```python
from build123d import *

# Parameters (mm, degrees)
LID_BLANK_DEPTH                 = 56
OUTER_PANEL_20DEG_DEPTH         = 143.098557347
OUTER_PANEL_20DEG_DEPTH_BACK    = 143.098557347
PANEL_3MM_DEPTH                 = 141.483885809
PANEL_3MM_DEPTH_BACK            = 141.483885809
HIDDEN_CASE_POST_0_START        = 3
SKETCH_4_R                      = 5
HIDDEN_CASE_POST_0_DEPTH        = 22.878191011
HIDDEN_CASE_POST_1_START        = 3
SKETCH_5_R                      = 5
HIDDEN_CASE_POST_1_DEPTH        = 22.878191011
HIDDEN_CASE_POST_2_START        = 3
SKETCH_6_R                      = 5
HIDDEN_CASE_POST_2_DEPTH        = 48.720077644
HIDDEN_CASE_POST_3_START        = 3
SKETCH_7_R                      = 5
HIDDEN_CASE_POST_3_DEPTH        = 48.720077644
FLUSH_OUTER_SURFACE_DEPTH       = 141.483885809
FLUSH_OUTER_SURFACE_DEPTH_BACK  = 141.483885809
BLIND_M3_0_START                = 3
SKETCH_9_R                      = 1.7
BLIND_M3_0_DEPTH                = 9.5
M3_SIDE_LOAD_NUT_0_START        = 3.1
SKETCH_10_W                     = 2.8
SKETCH_10_H                     = 5.8
M3_SIDE_LOAD_NUT_0_DEPTH        = 9.4
BLIND_M3_1_START                = 3
SKETCH_11_R                     = 1.7
BLIND_M3_1_DEPTH                = 9.5
M3_SIDE_LOAD_NUT_1_START        = 87.5
SKETCH_12_W                     = 2.8
SKETCH_12_H                     = 5.8
M3_SIDE_LOAD_NUT_1_DEPTH        = 9.4
BLIND_M3_2_START                = 3
SKETCH_13_R                     = 1.7
BLIND_M3_2_DEPTH                = 9.5
M3_SIDE_LOAD_NUT_2_START        = 3.1
SKETCH_14_W                     = 2.8
SKETCH_14_H                     = 5.8
M3_SIDE_LOAD_NUT_2_DEPTH        = 9.4
BLIND_M3_3_START                = 3
SKETCH_15_R                     = 1.7
BLIND_M3_3_DEPTH                = 9.5
M3_SIDE_LOAD_NUT_3_START        = 87.5
SKETCH_16_W                     = 2.8
SKETCH_16_H                     = 5.8
M3_SIDE_LOAD_NUT_3_DEPTH        = 9.4
SKETCH_17_R                     = 4.1
SHAFT_D8P2_DEPTH                = 5
SKETCH_18_W                     = 13.3
SKETCH_18_H                     = 13.3
BUTTON_13P3_CLEARANCE_DEPTH     = 5
SKETCH_19_R                     = 4
ENCODER_FRONT_BLIND_POST_DEPTH  = 11.07
ENCODER_FRONT_BLIND_SCREW_START = -14.07
SKETCH_20_R                     = 1.15
ENCODER_FRONT_BLIND_SCREW_DEPTH = 5
ENCODER_FRONT_M2_SIDE_NUT_START = 20.5
ENCODER_FRONT_M2_SIDE_NUT_DEPTH = 7.5
SKETCH_22_R                     = 4
ENCODER_REAR_BLIND_POST_DEPTH   = 11.07
ENCODER_REAR_BLIND_SCREW_START  = -14.07
SKETCH_23_R                     = 1.15
ENCODER_REAR_BLIND_SCREW_DEPTH  = 5
ENCODER_REAR_M2_SIDE_NUT_START  = 44.5
ENCODER_REAR_M2_SIDE_NUT_DEPTH  = 7.5
SKETCH_25_R                     = 4
BUTTON_LEFT_BLIND_POST_DEPTH    = 6.7
BUTTON_LEFT_BLIND_SCREW_START   = -9.7
SKETCH_26_R                     = 1.15
BUTTON_LEFT_BLIND_SCREW_DEPTH   = 5
BUTTON_LEFT_M2_SIDE_NUT_START   = 57.5
BUTTON_LEFT_M2_SIDE_NUT_DEPTH   = 7.5
SKETCH_28_R                     = 3.4
BUTTON_RIGHT_BLIND_POST_DEPTH   = 6.7
BUTTON_RIGHT_BLIND_SCREW_START  = -9.7
SKETCH_29_R                     = 1.15
BUTTON_RIGHT_BLIND_SCREW_DEPTH  = 5
BUTTON_RIGHT_M2_SIDE_NUT_START  = 90.8
BUTTON_RIGHT_M2_SIDE_NUT_DEPTH  = 7.5


with BuildPart() as part:
    # 草图1 → Lid_blank (new body)
    with BuildSketch(Plane.XY):
        with BuildLine():
            Line((6, 0), (94, 0))
            ThreePointArc((94, 0), (98.242640687, 1.757359313), (100, 6))
            Line((100, 6), (100, 78))
            ThreePointArc((100, 78), (98.242640687, 82.242640687), (94, 84))
            Line((94, 84), (6, 84))
            ThreePointArc((6, 84), (1.757359313, 82.242640687), (0, 78))
            Line((0, 78), (0, 6))
            ThreePointArc((0, 6), (1.757359313, 1.757359313), (6, 0))
        make_face()
    extrude(amount=LID_BLANK_DEPTH)

    # 草图2 → Outer_panel_20deg (cut, two sides: drawn at the far end of the back side and taken through both)
    with BuildSketch(Plane(origin=(0, 0, 0), x_dir=(0, 0, -1), z_dir=(1, 0, 0)).offset(-OUTER_PANEL_20DEG_DEPTH_BACK)):
        Polygon((-13.913128632, -20), (-61.229259087, 110), (-120, 110), (-120, -20), align=None)
    extrude(amount=OUTER_PANEL_20DEG_DEPTH + OUTER_PANEL_20DEG_DEPTH_BACK, mode=Mode.SUBTRACT)

    # 草图3 → Panel_3mm (cut, two sides: drawn at the far end of the back side and taken through both)
    with BuildSketch(Plane(origin=(0, 0, 0), x_dir=(0, 0, -1), z_dir=(1, 0, 0)).offset(-PANEL_3MM_DEPTH_BACK)):
        Polygon((-10.720595315, -20), (-58.036725769, 110), (30, 110), (30, -20), align=None)
    extrude(amount=PANEL_3MM_DEPTH + PANEL_3MM_DEPTH_BACK, mode=Mode.SUBTRACT)

    # 草图4 → Hidden_case_post_0 (add)
    with BuildSketch(Plane.XY.offset(HIDDEN_CASE_POST_0_START)):
        with Locations(Location((6.5, 6.5, 0), (0, 0, 270))):
            Circle(SKETCH_4_R)
    extrude(amount=HIDDEN_CASE_POST_0_DEPTH)

    # 草图5 → Hidden_case_post_1 (add)
    with BuildSketch(Plane.XY.offset(HIDDEN_CASE_POST_1_START)):
        with Locations(Location((93.5, 6.5, 0), (0, 0, 270))):
            Circle(SKETCH_5_R)
    extrude(amount=HIDDEN_CASE_POST_1_DEPTH)

    # 草图6 → Hidden_case_post_2 (add)
    with BuildSketch(Plane.XY.offset(HIDDEN_CASE_POST_2_START)):
        with Locations(Location((6.5, 77.5, 0), (0, 0, 270))):
            Circle(SKETCH_6_R)
    extrude(amount=HIDDEN_CASE_POST_2_DEPTH)

    # 草图7 → Hidden_case_post_3 (add)
    with BuildSketch(Plane.XY.offset(HIDDEN_CASE_POST_3_START)):
        with Locations(Location((93.5, 77.5, 0), (0, 0, 270))):
            Circle(SKETCH_7_R)
    extrude(amount=HIDDEN_CASE_POST_3_DEPTH)

    # 草图8 → Flush_outer_surface (cut, two sides: drawn at the far end of the back side and taken through both)
    with BuildSketch(Plane(origin=(0, 0, 0), x_dir=(0, 0, -1), z_dir=(1, 0, 0)).offset(-FLUSH_OUTER_SURFACE_DEPTH_BACK)):
        Polygon((-13.913128632, -20), (-61.229259087, 110), (-120, 110), (-120, -20), align=None)
    extrude(amount=FLUSH_OUTER_SURFACE_DEPTH + FLUSH_OUTER_SURFACE_DEPTH_BACK, mode=Mode.SUBTRACT)

    # 草图9 → Blind_M3_0 (cut)
    with BuildSketch(Plane.XY.offset(BLIND_M3_0_START)):
        with Locations((6.5, 6.5)):
            Circle(SKETCH_9_R)
    extrude(amount=BLIND_M3_0_DEPTH, mode=Mode.SUBTRACT)

    # 草图10 → M3_side_load_nut_0 (cut)
    with BuildSketch(Plane(origin=(0, 0, 0), x_dir=(0, 0, -1), z_dir=(1, 0, 0)).offset(M3_SIDE_LOAD_NUT_0_START)):
        with Locations((-6.4, 6.5)):
            Rectangle(SKETCH_10_W, SKETCH_10_H)
    extrude(amount=M3_SIDE_LOAD_NUT_0_DEPTH, mode=Mode.SUBTRACT)

    # 草图11 → Blind_M3_1 (cut)
    with BuildSketch(Plane.XY.offset(BLIND_M3_1_START)):
        with Locations((93.5, 6.5)):
            Circle(SKETCH_11_R)
    extrude(amount=BLIND_M3_1_DEPTH, mode=Mode.SUBTRACT)

    # 草图12 → M3_side_load_nut_1 (cut)
    with BuildSketch(Plane(origin=(0, 0, 0), x_dir=(0, 0, -1), z_dir=(1, 0, 0)).offset(M3_SIDE_LOAD_NUT_1_START)):
        with Locations((-6.4, 6.5)):
            Rectangle(SKETCH_12_W, SKETCH_12_H)
    extrude(amount=M3_SIDE_LOAD_NUT_1_DEPTH, mode=Mode.SUBTRACT)

    # 草图13 → Blind_M3_2 (cut)
    with BuildSketch(Plane.XY.offset(BLIND_M3_2_START)):
        with Locations((6.5, 77.5)):
            Circle(SKETCH_13_R)
    extrude(amount=BLIND_M3_2_DEPTH, mode=Mode.SUBTRACT)

    # 草图14 → M3_side_load_nut_2 (cut)
    with BuildSketch(Plane(origin=(0, 0, 0), x_dir=(0, 0, -1), z_dir=(1, 0, 0)).offset(M3_SIDE_LOAD_NUT_2_START)):
        with Locations((-6.4, 77.5)):
            Rectangle(SKETCH_14_W, SKETCH_14_H)
    extrude(amount=M3_SIDE_LOAD_NUT_2_DEPTH, mode=Mode.SUBTRACT)

    # 草图15 → Blind_M3_3 (cut)
    with BuildSketch(Plane.XY.offset(BLIND_M3_3_START)):
        with Locations((93.5, 77.5)):
            Circle(SKETCH_15_R)
    extrude(amount=BLIND_M3_3_DEPTH, mode=Mode.SUBTRACT)

    # 草图16 → M3_side_load_nut_3 (cut)
    with BuildSketch(Plane(origin=(0, 0, 0), x_dir=(0, 0, -1), z_dir=(1, 0, 0)).offset(M3_SIDE_LOAD_NUT_3_START)):
        with Locations((-6.4, 77.5)):
            Rectangle(SKETCH_16_W, SKETCH_16_H)
    extrude(amount=M3_SIDE_LOAD_NUT_3_DEPTH, mode=Mode.SUBTRACT)

    # 草图17 → Shaft_D8p2 (cut)
    with BuildSketch(Plane(origin=(0, -6.811148917, 18.71347785), x_dir=(1, 0, 0), z_dir=(0, -0.3420201433256689, 0.9396926207859084))):
        with Locations(Location((31, 44.248273283, 0), (0, 0, 270))):
            Circle(SKETCH_17_R)
    extrude(amount=-SHAFT_D8P2_DEPTH, mode=Mode.SUBTRACT)

    # 草图18 → Button_13p3_clearance (cut)
    with BuildSketch(Plane(origin=(0, -6.811148917, 18.71347785), x_dir=(1, 0, 0), z_dir=(0, -0.3420201433256689, 0.9396926207859084))):
        with Locations((77, 44.248273283)):
            Rectangle(SKETCH_18_W, SKETCH_18_H)
    extrude(amount=-BUTTON_13P3_CLEARANCE_DEPTH, mode=Mode.SUBTRACT)

    # 草图19 → Encoder_front_blind_post (add)
    with BuildSketch(Plane(origin=(0, -5.785088487, 15.894399988), x_dir=(-1, 0, 0), z_dir=(0, 0.34202014332566866, -0.9396926207859085))):
        with Locations(Location((-23, 30.748273283, 0), (0, 0, 270))):
            Circle(SKETCH_19_R)
    extrude(amount=ENCODER_FRONT_BLIND_POST_DEPTH)

    # 草图20 → Encoder_front_blind_screw (cut)
    with BuildSketch(Plane(origin=(0, -6.811148917, 18.71347785), x_dir=(1, 0, 0), z_dir=(0, -0.3420201433256689, 0.9396926207859084)).offset(ENCODER_FRONT_BLIND_SCREW_START)):
        with Locations(Location((23, 30.748273283, 0), (0, 0, 270))):
            Circle(SKETCH_20_R)
    extrude(amount=ENCODER_FRONT_BLIND_SCREW_DEPTH, mode=Mode.SUBTRACT)

    # 草图21 → Encoder_front_M2_side_nut (cut)
    with BuildSketch(Plane(origin=(0, 0, 0), x_dir=(0, 0, -1), z_dir=(1, 0, 0)).offset(ENCODER_FRONT_M2_SIDE_NUT_START)):
        Polygon((-17.169674452, 24.237605215), (-18.606159054, 28.184314222), (-20.297605771, 27.568677964), (-18.861121169, 23.621968957), align=None)
    extrude(amount=ENCODER_FRONT_M2_SIDE_NUT_DEPTH, mode=Mode.SUBTRACT)

    # 草图22 → Encoder_rear_blind_post (add)
    with BuildSketch(Plane(origin=(0, -5.785088487, 15.894399988), x_dir=(-1, 0, 0), z_dir=(0, 0.34202014332566866, -0.9396926207859085))):
        with Locations(Location((-47, 57.748273283, 0), (0, 0, 270))):
            Circle(SKETCH_22_R)
    extrude(amount=ENCODER_REAR_BLIND_POST_DEPTH)

    # 草图23 → Encoder_rear_blind_screw (cut)
    with BuildSketch(Plane(origin=(0, -6.811148917, 18.71347785), x_dir=(1, 0, 0), z_dir=(0, -0.3420201433256689, 0.9396926207859084)).offset(ENCODER_REAR_BLIND_SCREW_START)):
        with Locations(Location((47, 57.748273283, 0), (0, 0, 270))):
            Circle(SKETCH_23_R)
    extrude(amount=ENCODER_REAR_BLIND_SCREW_DEPTH, mode=Mode.SUBTRACT)

    # 草图24 → Encoder_rear_M2_side_nut (cut)
    with BuildSketch(Plane(origin=(0, 0, 0), x_dir=(0, 0, -1), z_dir=(1, 0, 0)).offset(ENCODER_REAR_M2_SIDE_NUT_START)):
        Polygon((-26.404218322, 49.609305976), (-27.840702923, 53.556014983), (-29.532149641, 52.940378725), (-28.095665039, 48.993669718), align=None)
    extrude(amount=ENCODER_REAR_M2_SIDE_NUT_DEPTH, mode=Mode.SUBTRACT)

    # 草图25 → Button_left_blind_post (add)
    with BuildSketch(Plane(origin=(0, -5.785088487, 15.894399988), x_dir=(-1, 0, 0), z_dir=(0, 0.34202014332566866, -0.9396926207859085))):
        with Locations(Location((-60, 25.248273283, 0), (0, 0, 270))):
            Circle(SKETCH_25_R)
    extrude(amount=BUTTON_LEFT_BLIND_POST_DEPTH)

    # 草图26 → Button_left_blind_screw (cut)
    with BuildSketch(Plane(origin=(0, -6.811148917, 18.71347785), x_dir=(1, 0, 0), z_dir=(0, -0.3420201433256689, 0.9396926207859084)).offset(BUTTON_LEFT_BLIND_SCREW_START)):
        with Locations(Location((60, 25.248273283, 0), (0, 0, 270))):
            Circle(SKETCH_26_R)
    extrude(amount=BUTTON_LEFT_BLIND_SCREW_DEPTH, mode=Mode.SUBTRACT)

    # 草图27 → Button_left_M2_side_nut (cut)
    with BuildSketch(Plane(origin=(0, 0, 0), x_dir=(0, 0, -1), z_dir=(1, 0, 0)).offset(BUTTON_LEFT_M2_SIDE_NUT_START)):
        Polygon((-19.395020416, 17.574667774), (-20.831505018, 21.521376781), (-22.522951736, 20.905740523), (-21.086467134, 16.959031516), align=None)
    extrude(amount=BUTTON_LEFT_M2_SIDE_NUT_DEPTH, mode=Mode.SUBTRACT)

    # 草图28 → Button_right_blind_post (add)
    with BuildSketch(Plane(origin=(0, -5.785088487, 15.894399988), x_dir=(-1, 0, 0), z_dir=(0, 0.34202014332566866, -0.9396926207859085))):
        with Locations(Location((-93.3, 45.248273283, 0), (0, 0, 270))):
            Circle(SKETCH_28_R)
    extrude(amount=BUTTON_RIGHT_BLIND_POST_DEPTH)

    # 草图29 → Button_right_blind_screw (cut)
    with BuildSketch(Plane(origin=(0, -6.811148917, 18.71347785), x_dir=(1, 0, 0), z_dir=(0, -0.3420201433256689, 0.9396926207859084)).offset(BUTTON_RIGHT_BLIND_SCREW_START)):
        with Locations(Location((93.3, 45.248273283, 0), (0, 0, 270))):
            Circle(SKETCH_29_R)
    extrude(amount=BUTTON_RIGHT_BLIND_SCREW_DEPTH, mode=Mode.SUBTRACT)

    # 草图30 → Button_right_M2_side_nut (cut)
    with BuildSketch(Plane(origin=(0, 0, 0), x_dir=(0, 0, -1), z_dir=(1, 0, 0)).offset(BUTTON_RIGHT_M2_SIDE_NUT_START)):
        Polygon((-26.235423283, 36.36852019), (-27.671907885, 40.315229197), (-29.363354602, 39.699592939), (-27.92687, 35.752883932), align=None)
    extrude(amount=BUTTON_RIGHT_M2_SIDE_NUT_DEPTH, mode=Mode.SUBTRACT)


solid = part.part
```
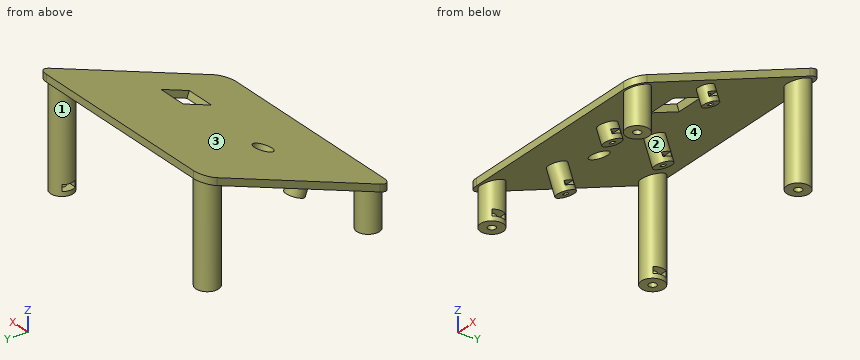
Part model, mm, in its own coordinate system. Face numbers are marked on the shaded views. A direction names the side the tool comes from. Round coordinates to 2 decimals unless told otherwise and drop trailing zeros. Loops run counter-clockwise (first coordinate to the right, second up) from the corner with the lowest first, then second, coordinate; pieces in that order, holes last.
Item 1: Cut at A-A, the plane z = 9. Give the cut face in (x, y), then the cut area to 3 significant figures.
Item 2: Cut at B-B, the plane x = 41.5. Give the cut face in (y, z).
Item 3: 3-axis set-ups, long thin cutter, end or side, ignore diameter. For the marked faces 1 and 2: which of +Z, -Z, +X, -X, +Y, -Y reach the whole face in a straight line?
Item 4: Drop flat-ended pins along their axis: P1, Ø10, axis at x = 44.5, y = 69.5, coming from the +Z side; P2, Ø2, axis at x = 6.5, y = 77.5, coming from the +Z side; P3, Ø3, axis at x = 8, z = 6, coming from the -Y side; P4, Ø10, axis at y = 50, z = 14, coming from the -X side (3 decimals). Give the stop position or say it passes through.
Item 5: Mould opens along Y. For the marked faces 3 and 4 say: +Y half, -Y half, draft (parallel to the pull), parting line (faces both ways), or undercut.
Item 6: Cut at C-C, the plane y = 59. Give the cut face in (x, z), then the cut area to 3 significant figures.
Item 7: Drill centre lines: line 1 (Y direction, x = 93.5, z = 10.4); line 2 (Y direction, x = 93, z = 9); line 3 (Z direction, x = 7.5, y = 76). Where is each one in solid material? Low to high.
A:
1. outline: circle Ø10 at (6.5, 6.5); circle Ø10 at (6.5, 77.5); circle Ø10 at (93.5, 6.5); circle Ø10 at (93.5, 77.5); hole circle Ø3.4 at (6.5, 6.5); hole circle Ø3.4 at (6.5, 77.5); hole circle Ø3.4 at (93.5, 6.5); hole circle Ø3.4 at (93.5, 77.5)
1. area: 278 mm2
2. outline: (0, 18) - (84, 48.57) - (84, 51.77) - (0, 21.19) - close
3. face 1: -Z
3. face 2: none
4. P1: stops at z = 48.31
4. P2: stops at z = 49.76
4. P3: stops at y = 1.5
4. P4: passes through
5. face 3: -Y half
5. face 4: undercut
6. outline: (0, 39.47) - (100, 39.47) - (100, 42.67) - (0, 42.67) - close
6. area: 319 mm2
7. line 1: y = 1.5 to 4.8, 8.2 to 11.5, 72.5 to 75.8, 79.2 to 82.5
7. line 2: y = 1.53 to 4.88, 8.12 to 11.47, 72.53 to 75.88, 79.12 to 82.47
7. line 3: z = 3 to 5, 7.8 to 48.85
